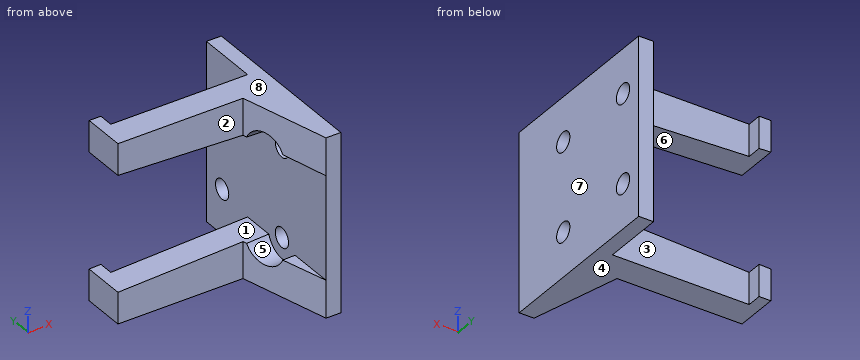
```python
from build123d import *

# Parameters (mm, degrees)
BOSS_EXTRUDE1_DEPTH     = 76.2
SKETCH2_W               = 70
SKETCH2_H               = 43.942
CUT_EXTRUDE1_DEPTH      = 76.2
SKETCH3_R               = 4.2164
CUT_EXTRUDE2_DEPTH      = 6.35
CUT_EXTRUDE2_DEPTH_BACK = 58.5
SKETCH3_3_R             = 8.89
SKETCH3_3_R_2           = 4.2164
CUT_EXTRUDE3_DEPTH      = 10


with BuildPart() as part:
    # Sketch1 → Boss-Extrude1 (new body)
    with BuildSketch(Plane.XY):
        Polygon((6.35, 0), (0, 0), (0, -26.2), (-58.5, -26.2), (-58.5, -19.85), (-63.5, -19.85), (-63.5, -38.2), (-10, -38.2), (0, -76.2), (6.35, -76.2), align=None)
    extrude(amount=BOSS_EXTRUDE1_DEPTH)

    # Sketch2 → Cut-Extrude1 (cut)
    with BuildSketch(Plane(origin=(0, 0, 0), x_dir=(1, 0, 0), z_dir=(0, 1, 0))):
        Polygon((0, -16.129), (0, -16.029), (-70, -13.129), (-70, -16.129), align=None)
        with Locations((-35, -38.1)):
            Rectangle(SKETCH2_W, SKETCH2_H)
        Polygon((0, -60.171), (-70, -63.071), (-70, -60.071), (0, -60.071), align=None)
    extrude(amount=-CUT_EXTRUDE1_DEPTH, mode=Mode.SUBTRACT)

    # Sketch3 → Cut-Extrude2 (cut, two sides)
    with BuildSketch(Plane(origin=(0, 0, 0), x_dir=(0, 0, -1), z_dir=(1, 0, 0))) as cut_extrude2_sk:
        with Locations((-19.05, -10)):
            Circle(SKETCH3_R)
        with Locations((-57.15, -10)):
            Circle(SKETCH3_R)
        with Locations((-57.15, -48.1)):
            Circle(SKETCH3_R)
        with Locations((-19.05, -48.1)):
            Circle(SKETCH3_R)
    extrude(amount=CUT_EXTRUDE2_DEPTH, mode=Mode.SUBTRACT)
    extrude(cut_extrude2_sk.sketch, amount=-CUT_EXTRUDE2_DEPTH_BACK, mode=Mode.SUBTRACT)

    # Sketch3<3> → Cut-Extrude3 (cut)
    with BuildSketch(Plane(origin=(0, 0, 0), x_dir=(0, 0, -1), z_dir=(1, 0, 0))):
        with Locations((-19.05, -48.1)):
            Circle(SKETCH3_3_R)
        with Locations((-19.05, -48.1)):
            Circle(SKETCH3_3_R_2, mode=Mode.SUBTRACT)
        with Locations((-57.15, -48.1)):
            Circle(SKETCH3_3_R)
        with Locations((-57.15, -48.1)):
            Circle(SKETCH3_3_R_2, mode=Mode.SUBTRACT)
    extrude(amount=-CUT_EXTRUDE3_DEPTH, mode=Mode.SUBTRACT)


solid = part.part
```
Source: CAD feature listing. Evaluate the final solid. Frame: model axes, mm. Face numbers are marked on the shaded views. A direction names the side the tool comes from. Give positions to 0.01 mm unless a question says otherwise; leave off trailing zeros. Loops run counter-clockwise (first coordinate to the right, second up) from the corner with the lowest first, then second, coordinate; pieces in that order, holes last. Notation, with made-up numbers: M 64.25,31 L 86.25,31 A34 ccw 86.25,64 Z; hole C 86.5,86 d6. An arc over 180 degrees is marked long. Put each result on its own line as item: value.
Q1. Section A-A (z = 57.15). Return the cut outline in (x, y).
Response values:
outline: M 0,-76.2 L 6.35,-76.2 L 6.35,-52.32 L 0,-52.32 Z; M 0,-43.88 L 6.35,-43.88 L 6.35,-14.22 L 0,-14.22 Z; M 0,-5.78 L 6.35,-5.78 L 6.35,0 L 0,0 Z
Q2. Reachability of the marked faces 1, 2, 3, 4 and 5 from +Z, -Z, +X, -X, +Y, -Y: full face, straight path, thin tool, end or side. Return the list, or none.
Response values:
face 1: -X, +Y, -Y
face 2: +Z, -Z, -X, -Y
face 3: +Z, -Z, +Y
face 4: -Z, +X, -X, +Y, -Y
face 5: -X
Q3. Pin query (flat end, axial travel): P1, Ø2.5, axis at x = -62, z = 67, coming from the +Y side; P2, Ø8, axis at y = -40.5, z = 26.5, coming from the -X side; P3, Ø8, axis at x = -40.5, z = 12, coming from the +Y side. Return the tip coordinate at first contact, or that it passes through.
Response values:
P1: stops at y = -19.85
P2: stops at x = 0
P3: stops at y = -26.2
Q4. Section C-C (y = -27.5). Return the cut outline in (x, z), and give its area (3 significant figures).
Response values:
outline: M -63.5,0 L 6.35,0 L 6.35,76.2 L -63.5,76.2 L -63.5,62.8 L 0,60.17 L 0,16.03 L -63.5,13.4 Z
area: 2,350 mm²
Q5. Line query: probe 1 along Y at (x, z) = (3, 57); probe 2 along X at (y, z) = (-57, 51); probe 3 along Y at (x, z) = (-36.5, 9). Output: solid intervals per line, ascending. Write a range as [from, to].
Response values:
probe 1: y = [-76.2, -52.31], [-43.89, -14.21], [-5.79, 0]
probe 2: x = [0, 6.35]
probe 3: y = [-38.2, -26.2]
Q6. Section D-D (x = -57). Return the cut outline in (y, z), and give its area (3 significant figures).
Response values:
outline: M -38.2,0 L -26.2,0 L -26.2,13.67 L -38.2,13.67 Z; M -38.2,62.53 L -26.2,62.53 L -26.2,76.2 L -38.2,76.2 Z
area: 328 mm²
Q7. Section B-B (y = -10). Return the cut outline in (x, z).
Response values:
outline: M 0,0 L 6.35,0 L 6.35,14.83 L 0,14.83 Z; M 0,23.27 L 6.35,23.27 L 6.35,52.93 L 0,52.93 Z; M 0,61.37 L 6.35,61.37 L 6.35,76.2 L 0,76.2 Z
Q8. Mould query, pull axis Z, two halves, no side actions, for the marked faces 6, 7 and 8. Classes: released by +Z, released by -Z, zero draft, split by the parting line, or undercut.
Response values:
face 6: undercut
face 7: zero draft
face 8: released by +Z
